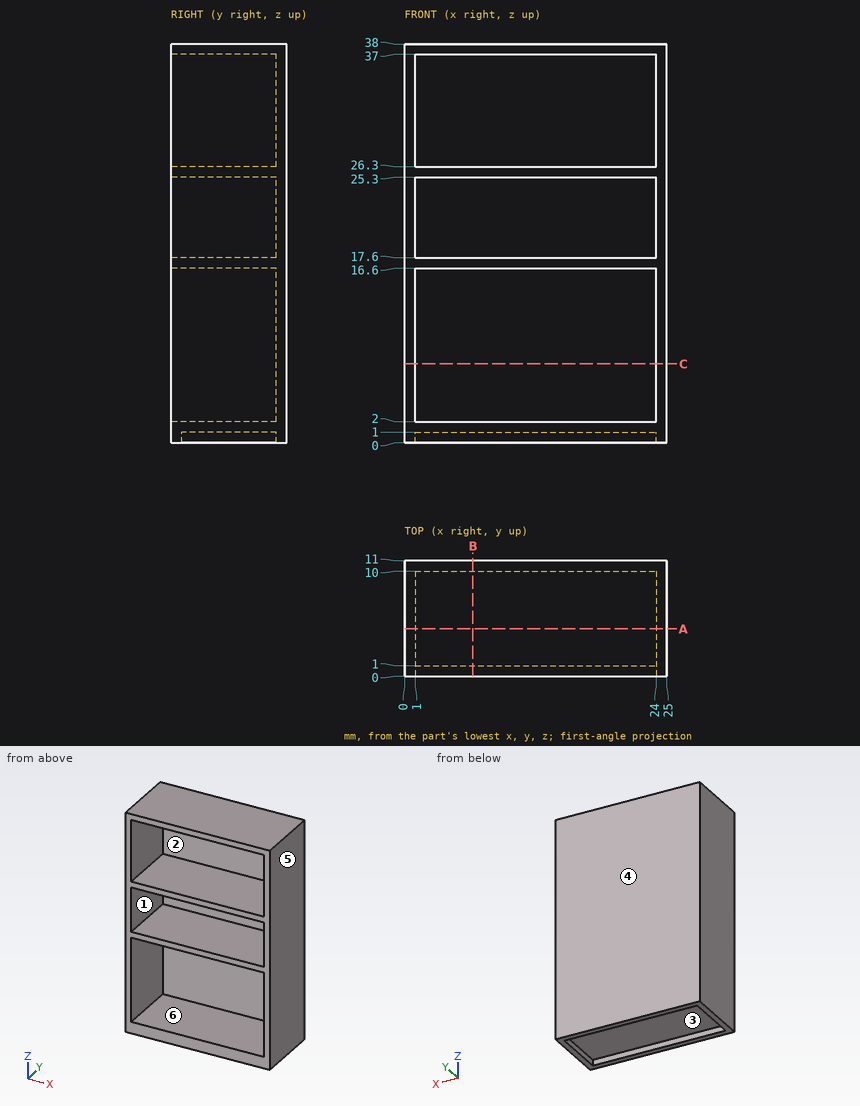
Input: dimensioned drawing with shaded views. Units: mm. Origin: part minimum x, y, z. A direction names the side the tool comes from. Give positions to 0.01 mm unless a question says otherwise; leave off trailing zeros. Write each loop counter-clockwise with the first axis right and the second up, starting at its lowest first coordinate (ties: lowest second). Pieces come first, ordered by that corner, then holes.
1. Access query for the marked faces 5 and 6. Directions: +Z, -Z, +X, -X, +Y, -Y. A direction counts if a zero-diameter tool reaches every point of the face in a straight line with its end or side. Return the directions, or none.
2. First-contact query: pin 1 (2.5 mm diameter, centred on x = 15, y = 6, fed in from -Z); pin 2 (3 mm diameter, centred on x = 8, z = 32, fed in from -Y). Flat tips, straight axial feed; report the tip coordinate or a pass-through.
3. Pull-direction query (Y, two-part tool) for the marked faces 1, 2, 3 and 4; classes: +Y half, -Y half, draft (parallel to the pull), parting line (faces both ways), or undercut.
4. Section query A-A (y = 4.5). Return the cut outline in (x, z), then the cut area to 3 significant figures.
5. Section query C-C (z = 7.5). Return the cut outline in (x, y).
6. Material intervals for line 1 along Z through (x, y) = (9, 5); line 2 along X through (y, z) = (5.25, 10.5); line 3 along Y through (x, z) = (9.75, 26.5), sorted ascending.
7. Section query B-B (x = 6.5). Return the cut outline in (y, z), then the cut area to 3 significant figures.
Output values:
1. face 5: +Z, -Z, +X, +Y, -Y
1. face 6: -Y
2. pin 1: stops at z = 1
2. pin 2: stops at y = 10
3. face 1: draft
3. face 2: -Y half
3. face 3: undercut
3. face 4: +Y half
4. outline: (0, 0) - (1, 0) - (1, 1) - (24, 1) - (24, 0) - (25, 0) - (25, 38) - (0, 38) - close; hole (1, 2) - (24, 2) - (24, 16.6) - (1, 16.6) - close; hole (1, 17.6) - (24, 17.6) - (24, 25.3) - (1, 25.3) - close; hole (1, 26.3) - (24, 26.3) - (24, 37) - (1, 37) - close
4. area: 168 mm2
5. outline: (0, 0) - (1, 0) - (1, 10) - (24, 10) - (24, 0) - (25, 0) - (25, 11) - (0, 11) - close
6. line 1: z = 1 to 2, 16.6 to 17.6, 25.3 to 26.3, 37 to 38
6. line 2: x = 0 to 1, 24 to 25
6. line 3: y = 10 to 11
7. outline: (0, 0) - (1, 0) - (1, 1) - (10, 1) - (10, 0) - (11, 0) - (11, 38) - (0, 38) - (0, 37) - (10, 37) - (10, 26.3) - (0, 26.3) - (0, 25.3) - (10, 25.3) - (10, 17.6) - (0, 17.6) - (0, 16.6) - (10, 16.6) - (10, 2) - (0, 2) - close
7. area: 79.0 mm2
